For this review, take the finished solid that the model builds, in its own axes (mm). A direction names the side the tool comes from. Coordinates: 2 decimals unless noted, no trailing zeros. Loops run counter-clockwise (first coordinate to the right, second up) from the corner with the lowest first, then second, coordinate; pieces in that order, holes last. Notation, with made-up numbers: M 6.25,-17.5 L 43.25,-17.5 A21 ccw 43.25,10.5 Z; hole C 64.25,-38.5 d7. An arc over 180 degrees is marked long. Answer as a JSON object with one key per item and string values. Group by question number.
Item 1: Add section A-A (x = 25.5). State the section outline as (y, z) points, then the cut area to 3 significant figures.
Item 2: Add section B-B (y = 4.9). Count the separate pieces of the cut face and the enclosed holes in it, then the cut area to 3 significant figures.
Item 3: Add section C-C (x = -1.5). State the section outline as (y, z) points.
Item 4: Tool access review of faces 1 (the face through (24, 3, 0.9)), 2 (the face through (59.89, 2.58, -0.92)), 3 (the face through (39.7, 5, -12)), 4 (the face through (-5.8, 3, 1)): name each direction out of +Z, -Z, +X, -X, +Y, -Y from which nothing blocks a thin tool from reaching the whole face with its end or side.
Item 5: Insertion check: pin 1 (0.5 mm diameter, centred on x = -6.5, y = 5, fed in from -Z); pin 2 (1.3 mm diameter, centred on x = 15.5, y = 5, fed in from +Z); pin 3 (0.8 mm diameter, centred on y = 4.5, z = -9, fed in from +X). Each pin has a flat end and moves straight along its axis. Give the tip position at first contact, or say it passes through.
Item 6: Wall thickness on L1, parallel to Z at x = 13, y = 5.3; L2, parallel to Z at x = -4, y = 2.75; L3, parallel to Z at x = 41.5, y = 3.6: over which ranges is each line inside the solid? List them lowest first. Write a range as from..to.
from build123d import *

# Parameters (mm, degrees)
EXTRUDE_1_DEPTH     = 4.2
EXTRUDE_START       = -1.6
EXTRUDE_2_DEPTH     = 1.6
CHAMFER_1_SIZE      = 2
CUT_EXTRUDE_1_DEPTH = 1.5
EXTRUDE_3_DEPTH     = 1.5
SKETCH_5_W          = 2.5
SKETCH_5_H          = 12.1
EXTRUDE_4_DEPTH     = 1.1
SKETCH_6_W          = 2
SKETCH_6_H          = 2
CUT_EXTRUDE_2_DEPTH = 69.191935007


with BuildPart() as part:
    # Эскиз1 → Бобышка-Вытянуть1 (new body)
    with BuildSketch(Plane(origin=(0, 1.5, 0), x_dir=(1, 0, 0), z_dir=(0, 1, 0))):
        with BuildLine():
            Line((46.05, -0.9), (-4.2, -0.9))
            Line((-4.2, -0.9), (-4.2, 1.1))
            Line((-4.2, 1.1), (-5.2, 1.1))
            Line((-5.2, 1.1), (-5.2, 4.95))
            Line((-5.2, 4.95), (-7.7, 4.95))
            Line((-7.7, 4.95), (-7.7, 3.95))
            Line((-7.7, 3.95), (-6.8, 3.95))
            Line((-6.8, 3.95), (-6.8, -0.5))
            Line((-6.8, -0.5), (-5.8, -0.5))
            Line((-5.8, -0.5), (-5.8, -2.5))
            Line((-5.8, -2.5), (46.05, -2.5))
            Line((46.05, -2.5), (50.55, -2.5))
            Line((50.55, -2.5), (51.5, -2.5))
            ThreePointArc((51.5, -2.5), (59.985281374, 1.014718626), (63.5, 9.5))
            Line((63.5, 9.5), (63.5, 21.5))
            ThreePointArc((63.5, 21.5), (62.621320344, 23.621320344), (60.5, 24.5))
            Line((60.5, 24.5), (-5.8, 24.5))
            Line((-5.8, 24.5), (-5.8, 22.5))
            Line((-5.8, 22.5), (-6.8, 22.5))
            Line((-6.8, 22.5), (-6.8, 18.05))
            Line((-6.8, 18.05), (-7.7, 18.05))
            Line((-7.7, 18.05), (-7.7, 17.05))
            Line((-7.7, 17.05), (-5.2, 17.05))
            Line((-5.2, 17.05), (-5.2, 20.9))
            Line((-5.2, 20.9), (-4.2, 20.9))
            Line((-4.2, 20.9), (-4.2, 22.9))
            Line((-4.2, 22.9), (60.5, 22.9))
            ThreePointArc((60.5, 22.9), (61.489949494, 22.489949494), (61.9, 21.5))
            Line((61.9, 21.5), (61.9, 9.5))
            ThreePointArc((61.9, 9.5), (58.853910524, 2.146089476), (51.5, -0.9))
            Line((51.5, -0.9), (50.55, -0.9))
            Line((50.55, -0.9), (46.05, -0.9))
        make_face()
    extrude(amount=EXTRUDE_1_DEPTH)

    # Эскиз2 → Бобышка-Вытянуть2 (add)
    with BuildSketch(Plane(origin=(0, 5.7, 0), x_dir=(1, 0, 0), z_dir=(0, 1, 0)).offset(EXTRUDE_START)):
        with BuildLine():
            Line((-7.7, 17.05), (-7.7, 4.95))
            Line((-7.7, 4.95), (-7.7, 3.95))
            Line((-7.7, 3.95), (-6.8, 3.95))
            Line((-6.8, 3.95), (-6.8, -0.5))
            Line((-6.8, -0.5), (-5.8, -0.5))
            Line((-5.8, -0.5), (-5.8, -2.5))
            Line((-5.8, -2.5), (51.5, -2.5))
            ThreePointArc((51.5, -2.5), (59.985281374, 1.014718626), (63.5, 9.5))
            Line((63.5, 9.5), (63.5, 21.5))
            ThreePointArc((63.5, 21.5), (62.621320344, 23.621320344), (60.5, 24.5))
            Line((60.5, 24.5), (-5.8, 24.5))
            Line((-5.8, 24.5), (-5.8, 22.5))
            Line((-5.8, 22.5), (-6.8, 22.5))
            Line((-6.8, 22.5), (-6.8, 18.05))
            Line((-6.8, 18.05), (-7.7, 18.05))
            Line((-7.7, 18.05), (-7.7, 17.05))
        make_face()
    extrude(amount=EXTRUDE_2_DEPTH)

    # Фаска1
    chamfer_1_edges = [part.edges().sort_by_distance(p)[0] for p in [
        (27.35, 5.7, -24.5),
        (62.621320344, 5.7, -23.621320344),
        (63.5, 5.7, -15.5),
        (59.985281374, 5.7, -1.014718626),
        (22.85, 5.7, 2.5),
    ]]
    chamfer(chamfer_1_edges, length=CHAMFER_1_SIZE)

    # Эскиз3 → Вырез-Вытянуть1 (cut)
    with BuildSketch(Plane(origin=(0, 5.7, 0), x_dir=(1, 0, 0), z_dir=(0, 1, 0))):
        with BuildLine():
            Line((0.570791566, 7.5), (-5.514169361, 1.291627678))
            ThreePointArc((-5.514169361, 1.291627678), (-5.72578868, 0.969696159), (-5.8, 0.591654733))
            Line((-5.8, 0.591654733), (-11.525705964, 0.591654733))
            Line((-11.525705964, 0.591654733), (-11.525705964, 21.408345267))
            Line((-11.525705964, 21.408345267), (-5.8, 21.408345267))
            ThreePointArc((-5.8, 21.408345267), (-5.72578868, 21.030303841), (-5.514169361, 20.708372322))
            Line((-5.514169361, 20.708372322), (0.570791566, 14.5))
            ThreePointArc((0.570791566, 14.5), (2, 11), (0.570791566, 7.5))
        make_face()
    extrude(amount=-CUT_EXTRUDE_1_DEPTH, mode=Mode.SUBTRACT)

    # Эскиз4 → Бобышка-Вытянуть3 (add)
    with BuildSketch(Plane.XZ.offset(-4.1)):
        with BuildLine():
            Line((-4.2, 0.9), (2.224149308, -8.093809031))
            ThreePointArc((2.224149308, -8.093809031), (3.155481952, -11), (2.224149308, -13.906190969))
            Line((2.224149308, -13.906190969), (-4.2, -22.9))
            Line((-4.2, -22.9), (-5.2, -22.9))
            Line((-5.2, -22.9), (-5.2, -17.05))
            Line((-5.2, -17.05), (-7.7, -17.05))
            Line((-7.7, -17.05), (-7.7, -4.95))
            Line((-7.7, -4.95), (-5.998027876, -4.95))
            Line((-5.998027876, -4.95), (-5.2, -1.1))
            Line((-5.2, -1.1), (-4.2, 0.9))
        make_face()
    extrude(amount=EXTRUDE_3_DEPTH)

    # Эскиз5 → Бобышка-Вытянуть4 (add)
    with BuildSketch(Plane.XZ.offset(-2.6)):
        with Locations((-6.45, -11)):
            Rectangle(SKETCH_5_W, SKETCH_5_H)
    extrude(amount=EXTRUDE_4_DEPTH)

    # Эскиз6 → Вырез-Вытянуть2 (cut, through all)
    with BuildSketch(Plane(origin=(0, 5.7, 0), x_dir=(1, 0, 0), z_dir=(0, 1, 0))):
        with Locations((18.7, 15)):
            Rectangle(SKETCH_6_W, SKETCH_6_H)
        with Locations((15.7, 15)):
            Rectangle(SKETCH_6_W, SKETCH_6_H)
        with Locations((12.7, 15)):
            Rectangle(SKETCH_6_W, SKETCH_6_H)
        with Locations((9.7, 15)):
            Rectangle(SKETCH_6_W, SKETCH_6_H)
        with Locations((18.7, 12)):
            Rectangle(SKETCH_6_W, SKETCH_6_H)
        with Locations((15.7, 12)):
            Rectangle(SKETCH_6_W, SKETCH_6_H)
        with Locations((12.7, 12)):
            Rectangle(SKETCH_6_W, SKETCH_6_H)
        with Locations((18.7, 9)):
            Rectangle(SKETCH_6_W, SKETCH_6_H)
        with Locations((15.7, 9)):
            Rectangle(SKETCH_6_W, SKETCH_6_H)
        with Locations((18.7, 6)):
            Rectangle(SKETCH_6_W, SKETCH_6_H)
        with Locations((32.7, 6)):
            Rectangle(SKETCH_6_W, SKETCH_6_H)
        with Locations((35.7, 9)):
            Rectangle(SKETCH_6_W, SKETCH_6_H)
        with Locations((32.7, 9)):
            Rectangle(SKETCH_6_W, SKETCH_6_H)
        with Locations((38.7, 12)):
            Rectangle(SKETCH_6_W, SKETCH_6_H)
        with Locations((35.7, 12)):
            Rectangle(SKETCH_6_W, SKETCH_6_H)
        with Locations((32.7, 12)):
            Rectangle(SKETCH_6_W, SKETCH_6_H)
        with Locations((41.7, 15)):
            Rectangle(SKETCH_6_W, SKETCH_6_H)
        with Locations((38.7, 15)):
            Rectangle(SKETCH_6_W, SKETCH_6_H)
        with Locations((35.7, 15)):
            Rectangle(SKETCH_6_W, SKETCH_6_H)
        with Locations((32.7, 15)):
            Rectangle(SKETCH_6_W, SKETCH_6_H)
    extrude(amount=-CUT_EXTRUDE_2_DEPTH, mode=Mode.SUBTRACT)


solid = part.part
From the geometry:
{
 "1": {"outline": "M 1.5,-24.5 L 3.7,-24.5 L 5.7,-22.5 L 5.7,0.5 L 3.7,2.5 L 1.5,2.5 L 1.5,0.9 L 4.1,0.9 L 4.1,-22.9 L 1.5,-22.9 Z", "area": "47.5 mm²"},
 "2": {"separate pieces": "1", "enclosed holes": "20", "area": "1,480 mm²"},
 "3": {"outline": "M 1.5,-24.5 L 3.7,-24.5 L 5.7,-22.5 L 5.7,-16.61 L 4.2,-16.61 L 4.2,-5.39 L 5.7,-5.39 L 5.7,0.5 L 3.7,2.5 L 1.5,2.5 L 1.5,0.9 L 4.1,0.9 L 4.1,-2.88 L 2.6,-2.88 L 2.6,-19.12 L 4.1,-19.12 L 4.1,-22.9 L 1.5,-22.9 Z"},
 "4": {"face 1": "-Y", "face 2": "+Z, +X, +Y, -Y", "face 3": "+Y, -Y", "face 4": "+Z, -X, +Y, -Y"},
 "5": {"pin 1": "stops at z = -22.5", "pin 2": "stops at z = 1.85", "pin 3": "stops at x = 63.09"},
 "6": {"L1": "z = -22.9..-16, -14..-13, -11..0.9", "L2": "z = -24.5..-22.9, -22.62..0.62, 0.9..2.5", "L3": "z = -24.5..-22.9, 0.9..2.5"}
}
